Model file for the job. Use its own axes, mm. Face numbers are marked on the shaded views. A direction names the side the tool comes from. Give positions to 0.01 mm unless a question says otherwise; leave off trailing zeros. Loops run counter-clockwise (first coordinate to the right, second up) from the corner with the lowest first, then second, coordinate; pieces in that order, holes last. Notation, with made-up numbers: M 76,85 L 126,85 A16 cw 126,114 Z; hole C 15,-12.5 d7. An arc over 180 degrees is marked long. Answer in a Markdown table with one row per item.
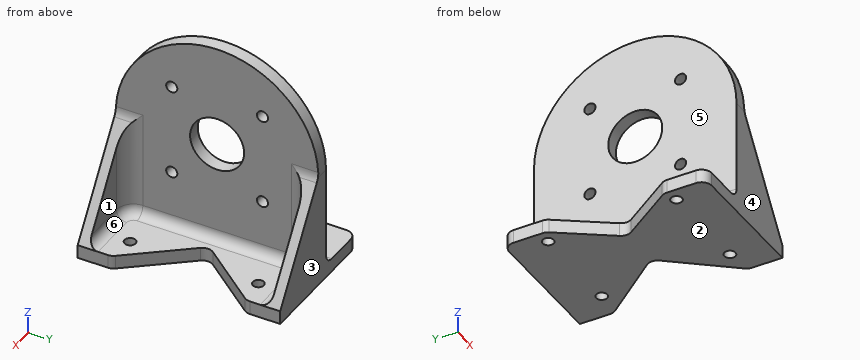
```python
from build123d import *

# Parameters (mm, degrees)
SKETCH_3_W          = 20
SKETCH_3_H          = 60
EXTRUDE_2_DEPTH     = 4
SKETCH_4_R          = 8
SKETCH_4_R_2        = 1.65
EXTRUDE_3_DEPTH     = 4
SKETCH_9_W          = 20
SKETCH_9_H          = 60
EXTRUDE_6_DEPTH     = 4
EXTRUDE_4_DEPTH     = 3
EXTRUDE_7_DEPTH     = 3
SKETCH_7_R          = 1.65
CUT_EXTRUDE_1_DEPTH = 74.484692283
FILLET_1_R          = 5
FILLET_2_R          = 3
FILLET_3_R          = 3


with BuildPart() as part:
    # 草图3 → 凸台-拉伸2 (new body)
    with BuildSketch(Plane.XY):
        Rectangle(SKETCH_3_W, SKETCH_3_H)
    extrude(amount=EXTRUDE_2_DEPTH)

    # 草图4 → 凸台-拉伸3 (add)
    with BuildSketch(Plane(origin=(10, 0, 0), x_dir=(0, 0, -1), z_dir=(1, 0, 0))):
        with BuildLine():
            Line((0, 30), (-34, 30))
            ThreePointArc((-34, 30), (-64, 0), (-34, -30))
            Line((-34, -30), (0, -30))
            Line((0, -30), (0, 30))
        make_face()
        with Locations(Location((-34, 0, 0), (0, 0, 90))):
            Circle(SKETCH_4_R, mode=Mode.SUBTRACT)
        with Locations(Location((-47.435028843, 13.435028843, 0), (0, 0, 90))):
            Circle(SKETCH_4_R_2, mode=Mode.SUBTRACT)
        with Locations(Location((-20.564971157, 13.435028843, 0), (0, 0, 270))):
            Circle(SKETCH_4_R_2, mode=Mode.SUBTRACT)
        with Locations(Location((-20.564971157, -13.435028843, 0), (0, 0, 90))):
            Circle(SKETCH_4_R_2, mode=Mode.SUBTRACT)
        with Locations(Location((-47.435028843, -13.435028843, 0), (0, 0, 270))):
            Circle(SKETCH_4_R_2, mode=Mode.SUBTRACT)
    extrude(amount=-EXTRUDE_3_DEPTH)

    # 草图9 → 凸台-拉伸6 (add)
    with BuildSketch(Plane.XY):
        with Locations((20, 0)):
            Rectangle(SKETCH_9_W, SKETCH_9_H)
    extrude(amount=EXTRUDE_6_DEPTH)

    # 草图5 → 凸台-拉伸4 (add)
    with BuildSketch(Plane(origin=(0, 30, 0), x_dir=(1, 0, 0), z_dir=(0, 1, 0))):
        Polygon((10, -34), (30, -4), (10, -4), align=None)
    extrude(amount=-EXTRUDE_4_DEPTH)

    # 草图11 → 凸台-拉伸7 (add)
    with BuildSketch(Plane.XZ.offset(30)):
        Polygon((10, 34), (10, 4), (30, 4), align=None)
    extrude(amount=-EXTRUDE_7_DEPTH)

    # 草图7 → 切除-拉伸1 (cut, through all)
    with BuildSketch(Plane.XY.offset(4)):
        with Locations((-6, 19)):
            Circle(SKETCH_7_R)
        with Locations((22, 19)):
            Circle(SKETCH_7_R)
        with Locations((22, -19)):
            Circle(SKETCH_7_R)
        with Locations((-6, -19)):
            Circle(SKETCH_7_R)
        Polygon((-10, 17.5), (2, 0), (-10, -17.5), align=None)
        Polygon((14, 0), (30, 20), (30, -20), align=None)
    extrude(amount=-CUT_EXTRUDE_1_DEPTH, mode=Mode.SUBTRACT)

    # 圆角1
    fillet_1_edges = [part.edges().sort_by_distance(p)[0] for p in [
        (10, 27, 19),
        (10, 28.5, 34),
        (10, -28.5, 34),
        (10, -27, 19),
    ]]
    fillet(fillet_1_edges, radius=FILLET_1_R)

    # 圆角2
    fillet_2_edges = [part.edges().sort_by_distance(p)[0] for p in [
        (-10, -17.5, 2),
        (-10, 17.5, 2),
        (2, 0, 2),
        (30, -20, 2),
        (14, 0, 2),
        (30, 20, 2),
        (10, 0, 4),
        (22.5, -27, 4),
        (11.464466094, 25.535533906, 4),
        (11.464466094, -25.535533906, 4),
        (22.5, 27, 4),
    ]]
    fillet(fillet_2_edges, radius=FILLET_2_R)

    # 圆角3
    fillet_3_edges = [part.edges().sort_by_distance(p)[0] for p in [
        (6, 0, 4),
        (-10, 30, 2),
        (-10, -30, 2),
    ]]
    fillet(fillet_3_edges, radius=FILLET_3_R)


solid = part.part
```
Q1. Mould opens along Y. For the marked faces 1, 2 and 3 say: released by +Y, released by -Y, zero draft, split by the parting line, or undercut.
Reported:
| item | result |
|---|---|
| face 1 | undercut |
| face 2 | zero draft |
| face 3 | released by +Y |
Q2. Saw through at A-A (y = 0). Give the cut face in (x, z), and give its area (3 significant figures).
Reported:
| item | result |
|---|---|
| outline | M 1.36,0 L 14.84,0 L 14.84,4 L 13,4 A3 cw 10,7 L 10,26 L 6,26 L 6,7 A3 cw 3,4 L 1.36,4 Z; M 6,42 L 10,42 L 10,64 L 6,64 Z |
| area | 234 mm² |
Q3. Drop flat-ended pins along their axis: pin 1 (8 mm diameter, centred on y = -8, z = 34, fed in from -X); pin 2 (4 mm diameter, centred on x = -1, y = 1.5, fed in from +Z); pin 3 (10 mm diameter, centred on x = 6.5, z = 42.5, fed in from -Y). Give the stop position or say it passes through.
Reported:
| item | result |
|---|---|
| pin 1 | x = 6 |
| pin 2 | z = 4 |
| pin 3 | y = -29.8 |
Q4. Saw through at B-B (x = 22). Give the cut face in (y, z).
Reported:
| item | result |
|---|---|
| outline | M -30,0 L -20.65,0 L -20.65,4 L -24,4 A3 cw -27,7 L -27,16 L -30,16 Z; M -17.35,0 L -10,0 L -10,4 L -17.35,4 Z; M 10,0 L 17.35,0 L 17.35,4 L 10,4 Z; M 20.65,0 L 30,0 L 30,16 L 27,16 L 27,7 A3 cw 24,4 L 20.65,4 Z |
Q5. Saw through at D-D (x = -6). Give the cut face in (y, z).
Reported:
| item | result |
|---|---|
| outline | M -30,0 L -20.65,0 L -20.65,4 L -30,4 Z; M -17.35,0 L -11.67,0 L -11.67,4 L -17.35,4 Z; M 11.67,0 L 17.35,0 L 17.35,4 L 11.67,4 Z; M 20.65,0 L 30,0 L 30,4 L 20.65,4 Z |
Q6. 3-axis set-ups, long thin cutter, end or side, ignore diameter. For the marked faces 4, 5 and 6: which of +Z, -Z, +X, -X, +Y, -Y reach the whole face in a straight line?
Reported:
| item | result |
|---|---|
| face 4 | +Z, -Z, +X, -X, -Y |
| face 5 | +Z, -X, +Y, -Y |
| face 6 | +Z, +X |
Q7. Saw through at C-C (z = 28.5). Give the cut face in (x, y).
Reported:
| item | result |
|---|---|
| outline | M 6,-30 L 13.67,-30 L 13.67,-26.82 A5 cw 10,-22 L 10,-5.81 L 6,-5.81 Z; M 6,5.81 L 10,5.81 L 10,22 A5 cw 13.67,26.82 L 13.67,30 L 6,30 Z |
Q8. Probe probe 1 along Y at (x, z) = (22, 1); probe 2 along Y at (x, z) = (-6, 1.65); probe 3 along X at (y, z) = (22, 12). List the from-to ranges inside material, lowest first.
Reported:
| item | result |
|---|---|
| probe 1 | -30 to -20.65, -17.35 to -10, 10 to 17.35, 20.65 to 30 |
| probe 2 | -30 to -20.65, -17.35 to -11.67, 11.67 to 17.35, 20.65 to 30 |
| probe 3 | 6 to 10 |
